Design review of the part built by this model. Coordinates are the model's own, in mm. Face numbers are marked on the shaded views. A direction names the side the tool comes from. Coordinates: 2 decimals unless noted, no trailing zeros. Loops run counter-clockwise (first coordinate to the right, second up) from the corner with the lowest first, then second, coordinate; pieces in that order, holes last. Notation, with made-up numbers: (41.25, 18) -> (76.25, 18) arc R20 cw to (76.25, 52) -> close; hole circle Ø1 at (51, 60). An arc over 180 degrees is marked (long way). Answer in a Markdown table with one row per item.
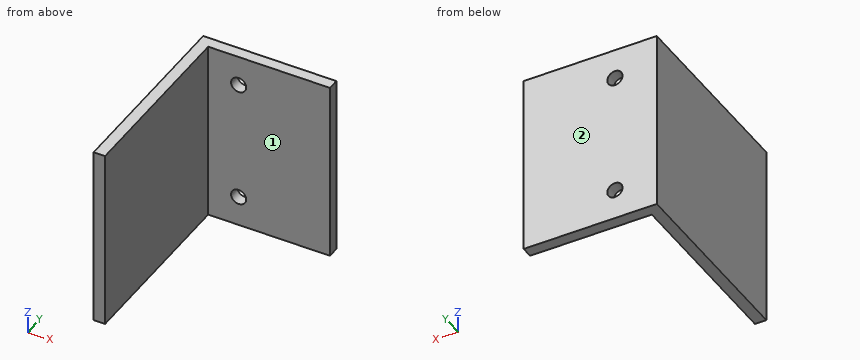
```python
from build123d import *

# Parameters (mm, degrees)
SKETCH1_W           = 35
SKETCH1_H           = 48
SKETCH1_R           = 2
BOSS_EXTRUDE1_DEPTH = 3
SKETCH2_W           = 3
SKETCH2_H           = 48
BOSS_EXTRUDE2_DEPTH = 48


with BuildPart() as part:
    # Sketch1 → Boss-Extrude1 (new body)
    with BuildSketch(Plane(origin=(0, 0, 0), x_dir=(1, 0, 0), z_dir=(0, 1, 0))):
        Rectangle(SKETCH1_W, SKETCH1_H)
        with Locations(Location((-6.5, 16, 0), (0, 0, 270))):
            Circle(SKETCH1_R, mode=Mode.SUBTRACT)
        with Locations(Location((-6.5, -16, 0), (0, 0, 90))):
            Circle(SKETCH1_R, mode=Mode.SUBTRACT)
    extrude(amount=BOSS_EXTRUDE1_DEPTH)

    # Sketch2 → Boss-Extrude2 (add)
    with BuildSketch(Plane.XZ):
        with Locations((-16, 0)):
            Rectangle(SKETCH2_W, SKETCH2_H)
    extrude(amount=BOSS_EXTRUDE2_DEPTH)


solid = part.part
```
(1) To check wall thickness, follow probe 1 along X at (y, z) = (1.4, -16); probe 2 along Z at (x, y) = (-6, 1); probe 3 along Y at (x, z) = (4.5, 14). State the ranges of each line that lie inside material, in increasing order.
Evaluation:
| item | result |
|---|---|
| probe 1 | x = -17.5 to -8.5, -4.5 to 17.5 |
| probe 2 | z = -24 to -17.94, -14.06 to 14.06, 17.94 to 24 |
| probe 3 | y = 0 to 3 |
(2) Take a section at C-C on y = -21. Give the boundary of the cut face in (x, z).
Evaluation:
| item | result |
|---|---|
| outline | (-17.5, -24) -> (-14.5, -24) -> (-14.5, 24) -> (-17.5, 24) -> close |
(3) Take a section at A-A on z = -16. Give the boundary of the cut face in (x, y), and give its area (3 significant figures).
Evaluation:
| item | result |
|---|---|
| outline | (-17.5, -48) -> (-14.5, -48) -> (-14.5, 0) -> (-8.5, 0) -> (-8.5, 3) -> (-17.5, 3) -> close; (-4.5, 0) -> (17.5, 0) -> (17.5, 3) -> (-4.5, 3) -> close |
| area | 237 mm² |
(4) Tool access review of the marked faces 1 and 2: name each direction out of +Z, -Z, +X, -X, +Y, -Y from which nothing blocks a thin tool from reaching the whole face with its end or side.
Evaluation:
| item | result |
|---|---|
| face 1 | +Z, -Z, +X, -Y |
| face 2 | +Z, -Z, +X, -X, +Y |
(5) For pin 1 (5 mm diameter, centred on x = -6.5, z = -16, fed in from +Y); pin 2 (5 mm diameter, centred on x = 9.5, z = -1.5, fed in from -Y), all flat-tipped, find the tip position at first contact; note any pin that passes through.
Evaluation:
| item | result |
|---|---|
| pin 1 | stops at y = 3 |
| pin 2 | stops at y = 0 |
(6) Take a section at D-D on x = 9. Give the boundary of the cut face in (y, z).
Evaluation:
| item | result |
|---|---|
| outline | (0, -24) -> (3, -24) -> (3, 24) -> (0, 24) -> close |
(7) Take a section at B-B on x = -6.5. Give the boundary of the cut face in (y, z).
Evaluation:
| item | result |
|---|---|
| outline | (0, -24) -> (3, -24) -> (3, -18) -> (0, -18) -> close; (0, -14) -> (3, -14) -> (3, 14) -> (0, 14) -> close; (0, 18) -> (3, 18) -> (3, 24) -> (0, 24) -> close |
